Geometry check sheet. Reference: the model listing, model coordinates, mm. A direction names the side the tool comes from. Round coordinates to 2 decimals unless told otherwise and drop trailing zeros. Loops run counter-clockwise (first coordinate to the right, second up) from the corner with the lowest first, then second, coordinate; pieces in that order, holes last.
```python
from build123d import *

# Parameters (mm, degrees)
SKETCH_1_W          = 25
SKETCH_1_H          = 34
EXTRUDE_1_DEPTH     = 1.2
SKETCH_1_3_W        = 0.7
SKETCH_1_3_H        = 2.5
SKETCH_1_3_R        = 0.635
CUT_EXTRUDE_1_DEPTH = 0.01
SKETCH_1_4_W        = 3
SKETCH_1_4_H        = 0.5
SKETCH_1_4_W_2      = 0.5
SKETCH_1_4_H_2      = 3
CUT_EXTRUDE_2_DEPTH = 2.2
FILLET_1_R          = 1
SKETCH_1_5_W        = 3.3
SKETCH_1_5_H        = 2
EXTRUDE_2_DEPTH     = 1.5


with BuildPart() as part:
    # Sketch 1 → Extrude 1 (new body)
    with BuildSketch(Plane.XY):
        with Locations((12.5, 17)):
            Rectangle(SKETCH_1_W, SKETCH_1_H)
    extrude(amount=-EXTRUDE_1_DEPTH)

    # Sketch 1_3 → Cut-Extrude 1 (cut)
    with BuildSketch(Plane.XY):
        with Locations((1.93, 28.778)):
            Rectangle(SKETCH_1_3_W, SKETCH_1_3_H)
        with Locations((3.2, 28.778)):
            Rectangle(SKETCH_1_3_W, SKETCH_1_3_H)
        with Locations((5.74, 28.778)):
            Rectangle(SKETCH_1_3_W, SKETCH_1_3_H)
        with Locations((7.01, 28.778)):
            Rectangle(SKETCH_1_3_W, SKETCH_1_3_H)
        with Locations((8.28, 28.778)):
            Rectangle(SKETCH_1_3_W, SKETCH_1_3_H)
        with Locations((13, 31.826)):
            Circle(SKETCH_1_3_R)
        with Locations((15.159, 31.826)):
            Circle(SKETCH_1_3_R)
        with Locations((4.47, 28.778)):
            Rectangle(SKETCH_1_3_W, SKETCH_1_3_H)
        with Locations((2.007, 9.787)):
            Rectangle(SKETCH_1_3_W, SKETCH_1_3_H)
        with Locations((3.277, 9.787)):
            Rectangle(SKETCH_1_3_W, SKETCH_1_3_H)
        with Locations((4.547, 9.787)):
            Rectangle(SKETCH_1_3_W, SKETCH_1_3_H)
        with Locations((5.817, 9.787)):
            Rectangle(SKETCH_1_3_W, SKETCH_1_3_H)
        with Locations((7.087, 9.787)):
            Rectangle(SKETCH_1_3_W, SKETCH_1_3_H)
        with Locations((8.357, 9.787)):
            Rectangle(SKETCH_1_3_W, SKETCH_1_3_H)
        with Locations((9.627, 9.787)):
            Rectangle(SKETCH_1_3_W, SKETCH_1_3_H)
        with Locations((10.897, 9.787)):
            Rectangle(SKETCH_1_3_W, SKETCH_1_3_H)
    extrude(amount=-CUT_EXTRUDE_1_DEPTH, mode=Mode.SUBTRACT)

    # Sketch 1_4 → Cut-Extrude 2 (cut, through all)
    with BuildSketch(Plane.XY):
        with Locations((10, 33.3)):
            Rectangle(SKETCH_1_4_W, SKETCH_1_4_H)
        with Locations((0.7, 12.5)):
            Rectangle(SKETCH_1_4_W_2, SKETCH_1_4_H_2)
        with Locations((24.3, 12.5)):
            Rectangle(SKETCH_1_4_W_2, SKETCH_1_4_H_2)
    extrude(amount=-CUT_EXTRUDE_2_DEPTH, mode=Mode.SUBTRACT)

    # Fillet 1
    fillet_1_edges = [part.edges().sort_by_distance(p)[0] for p in [
        (0, 0, -0.6),
        (0, 34, -0.6),
        (25, 34, -0.6),
        (25, 0, -0.6),
    ]]
    fillet(fillet_1_edges, radius=FILLET_1_R)

    # Sketch 1_5 → Extrude 2 (add)
    with BuildSketch(Plane.XY):
        with Locations((21.4, 25)):
            Rectangle(SKETCH_1_5_W, SKETCH_1_5_H)
        with Locations((21.4, 22.86)):
            Rectangle(SKETCH_1_5_W, SKETCH_1_5_H)
    extrude(amount=EXTRUDE_2_DEPTH)


solid = part.part
```
1) Sectioned sample at A-A, the plane y = 11.5. Record the cut outline in (x, z), then the cut area to 3 significant figures.
Report:
outline: (0, -1.2) - (0.45, -1.2) - (0.45, 0) - (0, 0) - close; (0.95, -1.2) - (24.05, -1.2) - (24.05, 0) - (0.95, 0) - close; (24.55, -1.2) - (25, -1.2) - (25, 0) - (24.55, 0) - close
area: 28.8 mm2
2) Mould release check, pull along Y, two halves, no side actions. Record for faces 4 (the face through (10, 33.05, -1)), 5 (the face through (21, 21.86, 1)), 6 (the face through (21, 26, 1)), 7 (the face through (0.45, 12, -1)): +Y half, -Y half, draft (parallel to the pull), parting line (faces both ways), or undercut.
Report:
face 4: undercut
face 5: -Y half
face 6: +Y half
face 7: undercut
3) Sectioned sample at C-C, the plane y = 16. Record the cut outline in (x, z).
Report:
outline: (0, -1.2) - (25, -1.2) - (25, 0) - (0, 0) - close
4) Access from +Z, -Z, +X, -X, +Y, -Y to the whole of each face (thin tool, end or side, straight path). Record for faces 1 (the face through (12, 0, -1)), 2 (the face through (24.55, 12, -1)), 3 (the face through (23.05, 23, 1)).
Report:
face 1: +Z, -Z, +X, -X, -Y
face 2: +Z, -Z
face 3: +Z, +X, +Y, -Y
5) Gauge pin test, flat ends, axial feed: pin 1 (1.5 mm diameter, centred on x = 5, z = 1, fed in from -Y); pin 2 (1.6 mm diameter, centred on y = 22.5, z = 1, fed in from -X). Record the tip position at first contact, or that the pin passes through.
Report:
pin 1: passes through
pin 2: stops at x = 19.75
6) Scan lines: line 1 along Z through (x, y) = (12.5, 29); line 2 along Y through (x, z) = (9.5, -0.05); line 3 along X through (y, z) = (23.5, 1.15). Record each from-to range of solid material in increasing order.
Report:
line 1: z = -1.2 to 0
line 2: y = 0 to 33.05, 33.55 to 34
line 3: x = 19.75 to 23.05
